Geometry check sheet. Reference: the model listing, model coordinates, mm. Face numbers are marked on the shaded views. A direction names the side the tool comes from. Give positions to 0.01 mm unless a question says otherwise; leave off trailing zeros. Order: outer loops, then holes, each group sorted by start corner. A loop starts at its lowest first (then second) coordinate and runs counter-clockwise, first axis right, second up. Notation, with made-up numbers: (9, 42.25) - (47, 42.25) arc R22 cw to (47, 77.25) - close; hole circle Ø8 at (48.5, -21.75). An arc over 180 degrees is marked (long way). Put each result on its own line as item: value. Start each with the question number.
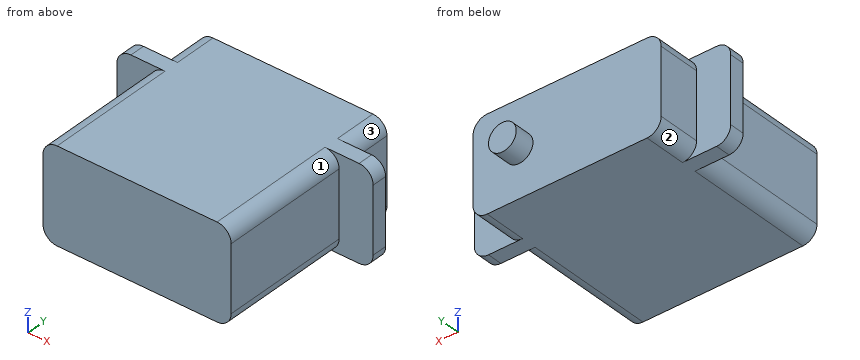
```python
from build123d import *

# Parameters (mm, degrees)
SKETCH1_W           = 40
SKETCH1_H           = 20
BOSS_EXTRUDE1_DEPTH = 40
SKETCH2_W           = 54.5
SKETCH2_H           = 3.2
BOSS_EXTRUDE2_DEPTH = 20
FILLET1_R           = 3
SKETCH3_R           = 2.95
BOSS_EXTRUDE3_DEPTH = 4.3


with BuildPart() as part:
    # Sketch1 → Boss-Extrude1 (new body)
    with BuildSketch(Plane(origin=(0, 0, 0), x_dir=(1, 0, 0), z_dir=(0, 1, 0))):
        Rectangle(SKETCH1_W, SKETCH1_H)
    extrude(amount=BOSS_EXTRUDE1_DEPTH)

    # Sketch2 → Boss-Extrude2 (add)
    with BuildSketch(Plane.XY.offset(10)):
        with Locations((0, 29.3)):
            Rectangle(SKETCH2_W, SKETCH2_H)
    extrude(amount=-BOSS_EXTRUDE2_DEPTH)

    # Fillet1
    fillet1_edges = [part.edges().sort_by_distance(p)[0] for p in [
        (20, 13.85, 10),
        (-20, 13.85, 10),
        (-20, 13.85, -10),
        (20, 13.85, -10),
        (27.25, 29.3, 10),
        (27.25, 29.3, -10),
        (-27.25, 29.3, -10),
        (-27.25, 29.3, 10),
        (20, 35.45, 10),
        (-20, 35.45, 10),
        (-20, 35.45, -10),
        (20, 35.45, -10),
    ]]
    fillet(fillet1_edges, radius=FILLET1_R)

    # Sketch3 → Boss-Extrude3 (add)
    with BuildSketch(Plane(origin=(0, 40, 0), x_dir=(1, 0, 0), z_dir=(0, 1, 0))):
        with Locations(Location((10.2, 0, 0), (0, 0, 90))):
            Circle(SKETCH3_R)
    extrude(amount=BOSS_EXTRUDE3_DEPTH)


solid = part.part
```
Item 1: Gauge pin test, flat ends, axial feed: pin 1 Ø3 at (x, z) = (20, 1) entering from +Y; pin 2 Ø5 at (x, y) = (-21, 5.5) entering from +Z; pin 3 Ø5 at (y, z) = (4.5, -4) entering from -X; pin 4 Ø1 at (x, z) = (-15.5, -0.5) entering from -Y. Record the tip position at first contact, or that the pin passes through.
Item 2: Cross-section at B-B (z = 6). Enter the section's corners in (x, y), and give its area (3 significant figures).
Item 3: Cross-section at A-A (x = 10.2). Enter the section's corners in (y, z).
Item 4: Set-up check for the marked faces 1, 2 and 3: record each of +Z, -Z, +X, -X, +Y, -Y from which the full face is reachable in a straight line by a thin tool's end or side.
Item 5: Cross-section at D-D (z = -2). Enter the section's corners in (x, y), and give its area (3 significant figures).
Item 6: Cross-section at C-C (y = 39). Enter the section's corners in (x, z), and give its area (3 significant figures).
Item 7: Thickness scan on line 1 along Y through (x, z) = (10, -5); line 2 along Y through (x, z) = (25, -9); line 3 along X through (y, z) = (12, 0.5). Record the ranges inside material, lowest first.
Recorded:
1. pin 1: stops at y = 40
1. pin 2: stops at z = 9.6
1. pin 3: stops at x = -20
1. pin 4: stops at y = 0
2. outline: (-27.25, 27.7) - (-20, 27.7) - (-20, 0) - (20, 0) - (20, 27.7) - (27.25, 27.7) - (27.25, 30.9) - (20, 30.9) - (20, 40) - (-20, 40) - (-20, 30.9) - (-27.25, 30.9) - close
2. area: 1,650 mm^2
3. outline: (0, -10) - (40, -10) - (40, -2.95) - (44.3, -2.95) - (44.3, 2.95) - (40, 2.95) - (40, 10) - (0, 10) - close
4. face 1: +Z, +X, -Y
4. face 2: -Z, -X, +Y
4. face 3: +Z, +X, +Y
5. outline: (-27.25, 27.7) - (-20, 27.7) - (-20, 0) - (20, 0) - (20, 27.7) - (27.25, 27.7) - (27.25, 30.9) - (20, 30.9) - (20, 40) - (12.37, 40) - (12.37, 44.3) - (8.03, 44.3) - (8.03, 40) - (-20, 40) - (-20, 30.9) - (-27.25, 30.9) - close
5. area: 1,670 mm^2
6. outline: (-20, -7) arc R3 ccw to (-17, -10) - (17, -10) arc R3 ccw to (20, -7) - (20, 7) arc R3 ccw to (17, 10) - (-17, 10) arc R3 ccw to (-20, 7) - close
6. area: 792 mm^2
7. line 1: y = 0 to 40
7. line 2: y = 27.7 to 30.9
7. line 3: x = -20 to 20
